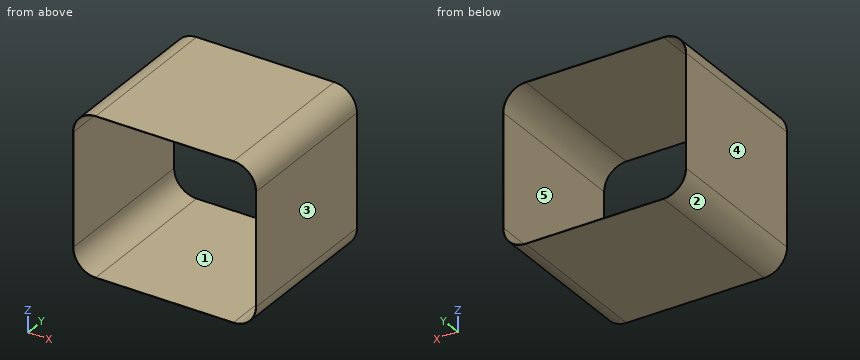
```python
from build123d import *

# Parameters (mm, degrees)
BOSS_EXTRUDE1_DEPTH = 1397
SHELL1_T            = -2.54
CUT_EXTRUDE3_REACH  = 4.54


with BuildPart() as part:
    # Sketch1 → Boss-Extrude1 (new body)
    with BuildSketch(Plane(origin=(0, 0, 0), x_dir=(1, 0, 0), z_dir=(0, 1, 0))):
        with BuildLine():
            Line((-203.2, -406.4), (1028.7, -406.4))
            ThreePointArc((1028.7, -406.4), (1172.384097937, -346.884097937), (1231.9, -203.2))
            Line((1231.9, -203.2), (1231.9, 800.1))
            ThreePointArc((1231.9, 800.1), (1172.384097937, 943.784097937), (1028.7, 1003.3))
            Line((1028.7, 1003.3), (-203.2, 1003.3))
            ThreePointArc((-203.2, 1003.3), (-346.884097937, 943.784097937), (-406.4, 800.1))
            Line((-406.4, 800.1), (-406.4, -203.2))
            ThreePointArc((-406.4, -203.2), (-346.884097937, -346.884097937), (-203.2, -406.4))
        make_face()
    extrude(amount=BOSS_EXTRUDE1_DEPTH)

    # Shell1
    shell1_openings = [part.faces().sort_by_distance(p)[0] for p in [
        (412.75, 0, -298.45),
    ]]
    offset(amount=SHELL1_T, openings=shell1_openings, kind=Kind.INTERSECTION)

    # Sketch3 → Cut-Extrude3 (cut, up to next)
    with BuildSketch(Plane.XZ.offset(-1394.46), mode=Mode.PRIVATE) as cut_extrude3_sk1:
        with BuildLine():
            Line((-403.86, 203.2), (-403.86, -800.1))
            ThreePointArc((-403.86, -800.1), (-345.088046713, -941.988046713), (-203.2, -1000.76))
            Line((-203.2, -1000.76), (1028.7, -1000.76))
            ThreePointArc((1028.7, -1000.76), (1170.588046713, -941.988046713), (1229.36, -800.1))
            Line((1229.36, -800.1), (1229.36, 203.2))
            ThreePointArc((1229.36, 203.2), (1170.588046713, 345.088046713), (1028.7, 403.86))
            Line((1028.7, 403.86), (-203.2, 403.86))
            ThreePointArc((-203.2, 403.86), (-345.088046713, 345.088046713), (-403.86, 203.2))
        make_face()
    cut_extrude3_tool1 = extrude(cut_extrude3_sk1.sketch, amount=-CUT_EXTRUDE3_REACH, mode=Mode.PRIVATE) & part.part
    add(cut_extrude3_tool1.solids().sort_by_distance((412.75, 1394.46, -298.45))[0], mode=Mode.SUBTRACT)


solid = part.part
```
Here's how the part is built. I have some questions about the finished solid (model axes, mm). Face numbers are marked on the shaded views. A direction names the side the tool comes from. Round coordinates to 2 decimals unless told otherwise and drop trailing zeros. Write each loop counter-clockwise with the first axis right and the second up, starting at its lowest first coordinate (ties: lowest second). Pieces come first, ordered by that corner, then holes. Notation, with made-up numbers: M 19.25,45.25 L 27.25,45.25 A13 cw 27.25,52.25 Z; hole C 16,-12.5 d9. An arc over 180 degrees is marked long. Answer as CSV lines item,"result". Start each with the question number.
1. I need wall thicknesses on probe 1 along Z at (x, y) = (159, 780); probe 2 along X at (y, z) = (142, -789.5); probe 3 along X at (y, z) = (1227.5, 264). Which ranges of each line are inside material? Lowest first, please.
2. Suppose I cut it at B-B on x = 122. Write out the boundary of the cut face in (y, z), then the cut area to 3 significant figures.
3. Suppose I cut it at C-C on y = 1248. Write out the boundary of the cut face in (x, z), then the cut area to 3 significant figures.
4. Thinking about a two-plate mould opening in Z: for the marked faces 1, 2 and 3, which applies, released by +Z, released by -Z, zero draft, split by the parting line, or undercut?
5. Suppose I cut it at A-A on z = -276.5. Write out the boundary of the cut face in (x, y).
6. On a 3-axis mill with a long thin cutter (end or side, diameter ignored), from which of +Z, -Z, +X, -X, +Y, -Y can I reach the whole of each face in a straight line? I mean the marked faces 4 and 5. Say none if no direction works.
Check result:
1,probe 1,"z = -1003.3 to -1000.76, 403.86 to 406.4"
1,probe 2,"x = -406.4 to -403.86, 1229.36 to 1231.9"
1,probe 3,"x = -397.09 to -394.43, 1219.93 to 1222.59"
2,outline,"M 0,-1003.3 L 1397,-1003.3 L 1397,-1000.76 L 0,-1000.76 Z; M 0,403.86 L 1397,403.86 L 1397,406.4 L 0,406.4 Z"
2,area,"7,100 mm2"
3,outline,"M -406.4,-800.1 A203.2 ccw -203.2,-1003.3 L 1028.7,-1003.3 A203.2 ccw 1231.9,-800.1 L 1231.9,203.2 A203.2 ccw 1028.7,406.4 L -203.2,406.4 A203.2 ccw -406.4,203.2 Z; hole M -403.86,-800.1 A200.66 ccw -203.2,-1000.76 L 1028.7,-1000.76 A200.66 ccw 1229.36,-800.1 L 1229.36,203.2 A200.66 ccw 1028.7,403.86 L -203.2,403.86 A200.66 ccw -403.86,203.2 Z"
3,area,"14,600 mm2"
4,face 1,"undercut"
4,face 2,"released by -Z"
4,face 3,"zero draft"
5,outline,"M -406.4,0 L -403.86,0 L -403.86,1397 L -406.4,1397 Z; M 1229.36,0 L 1231.9,0 L 1231.9,1397 L 1229.36,1397 Z"
6,face 4,"+Z, -Z, -X, +Y, -Y"
6,face 5,"+Y, -Y"
